Part model, mm, in its own coordinate system. A direction names the side the tool comes from. Round coordinates to 2 decimals unless told otherwise and drop trailing zeros. Order: outer loops, then holes, each group sorted by start corner. A loop starts at its lowest first (then second) coordinate and runs counter-clockwise, first axis right, second up. Notation, with made-up numbers: (25.5, 14.5) -> (49.5, 14.5) arc R14 ccw to (49.5, 23.5) -> close; hole circle Ø10 at (53, -12). An arc over 180 degrees is marked (long way). Answer as a JSON object with one key per item and string values. Group by question number.
```python
from build123d import *

# Parameters (mm, degrees)
SKETCH1_R             = 2.6
BOSS_EXTRUDE1_DEPTH   = 1.6
SKETCH2_R             = 3.45
BOSS_EXTRUDE2_DEPTH   = 1.4
M5X0_8_TAPPED_HOLE1_D = 4.2


with BuildPart() as part:
    # Sketch1 → Boss-Extrude1 (new body)
    with BuildSketch(Plane.XY):
        with BuildLine():
            Line((-10, -8.5), (-10, 8.5))
            ThreePointArc((-10, 8.5), (-9.560660172, 9.560660172), (-8.5, 10))
            Line((-8.5, 10), (-5, 10))
            Line((-5, 10), (-5, 37.485))
            Line((-5, 37.485), (-3.841886117, 40.959341649))
            ThreePointArc((-3.841886117, 40.959341649), (-3.295926597, 41.701863278), (-2.41886117, 41.985))
            Line((-2.41886117, 41.985), (2.41886117, 41.985))
            ThreePointArc((2.41886117, 41.985), (3.295926597, 41.701863278), (3.841886117, 40.959341649))
            Line((3.841886117, 40.959341649), (5, 37.485))
            Line((5, 37.485), (5, 10))
            Line((5, 10), (8.5, 10))
            ThreePointArc((8.5, 10), (9.560660172, 9.560660172), (10, 8.5))
            Line((10, 8.5), (10, -8.5))
            ThreePointArc((10, -8.5), (9.560660172, -9.560660172), (8.5, -10))
            Line((8.5, -10), (5, -10))
            Line((5, -10), (5, -37.485))
            Line((5, -37.485), (3.841886117, -40.959341649))
            ThreePointArc((3.841886117, -40.959341649), (3.295926597, -41.701863278), (2.41886117, -41.985))
            Line((2.41886117, -41.985), (-2.41886117, -41.985))
            ThreePointArc((-2.41886117, -41.985), (-3.295926597, -41.701863278), (-3.841886117, -40.959341649))
            Line((-3.841886117, -40.959341649), (-5, -37.485))
            Line((-5, -37.485), (-5, -10))
            Line((-5, -10), (-8.5, -10))
            ThreePointArc((-8.5, -10), (-9.560660172, -9.560660172), (-10, -8.5))
        make_face()
        Circle(SKETCH1_R, mode=Mode.SUBTRACT)
    extrude(amount=BOSS_EXTRUDE1_DEPTH)

    # Sketch2 → Boss-Extrude2 (add)
    with BuildSketch(Plane.XY.offset(1.6)):
        with Locations((0, 14.95)):
            Circle(SKETCH2_R)
        with Locations((0, 34.95)):
            Circle(SKETCH2_R)
        with Locations((0, -14.95)):
            Circle(SKETCH2_R)
        with Locations((0, -34.95)):
            Circle(SKETCH2_R)
    extrude(amount=BOSS_EXTRUDE2_DEPTH)

    # M5x0.8 Tapped Hole1 (through all)
    with Locations(Plane.XY.offset(3)):
        with Locations((0, 34.95), (0, 14.95), (0, -14.95), (0, -34.95)):
            Hole(M5X0_8_TAPPED_HOLE1_D / 2)


solid = part.part
```
Q1. Band-saw the part on B-B (y = -34.95). List the corners of the cut face in (x, z).
Q2. Wall check: line 1 (Y direction, x = 0, z = 0.7) (3 decimals); line 2 (X direction, y = 35, z = 0.1); line 3 (Z direction, x = 3.25, y = 19.5). Give the ranges that are in metal, low to high. Write a range as [from, to].
Q3. Drop flat-ended pins along their axis: pin 1 Ø4 at (x, y) = (0, 0) entering from +Z; pin 2 Ø10 at (x, y) = (-3.5, 4.5) entering from +Z; pin 3 Ø0.5 at (x, z) = (6.5, 1) entering from +Y; pin 4 Ø0.8 at (y, z) = (-29.5, 1) entering from -X. Give the stop position or say it passes through.
Q4. Band-saw the part on A-A (z = 2.45). List the corners of the cut face in (x, y), plus the area to 3 significant figures.
Q5. Band-saw the part on C-C (x = 6.5). List the corners of the cut face in (y, z).
Q6. Which spindle directions (+Z, -Z, +X, -X, +Y, -Y) get a long thin tool onto all of the face, cutting with end or side? Do faces 1 (the flat face through (-0.05, -17.2, 3)), 2 (the flat face through (-7, -10, 1)), 3 (the flat face through (7, -10, 1)), 4 (the flat face through (7, 10, 1)), 5 (the cylindrical face through (-0.45, 38.37, 2.29)). Say none if no direction does.
Q7. Two-plate mould, pull along Y, no slides. Class faces 6 (the cylindrical face through (-0.338, 2.578, 0.789)), 7 (the cylindrical face through (-1.13, 16.72, 1.48)), 8 (the cylindrical face through (9.55, 9.57, 0.79)), 9 (the flat face through (-5, -24, 1)): +Y half, -Y half, draft (parallel to the pull), parting line (faces both ways), or undercut.
Q8. Band-saw the part on D-D (y = 0). List the corners of the cut face in (x, z).
Completed:
{
 "1": {"outline": "(-5, 0) -> (-2.1, 0) -> (-2.1, 3) -> (-3.45, 3) -> (-3.45, 1.6) -> (-5, 1.6) -> close; (2.1, 0) -> (5, 0) -> (5, 1.6) -> (3.45, 1.6) -> (3.45, 3) -> (2.1, 3) -> close"},
 "2": {"line 1": "[-41.985, -37.05], [-32.85, -17.05], [-12.85, -2.6], [2.6, 12.85], [17.05, 32.85], [37.05, 41.985]", "line 2": "[-5, -2.1], [2.1, 5]", "line 3": "[0, 1.6]"},
 "3": {"pin 1": "through", "pin 2": "z = 1.6", "pin 3": "y = 10", "pin 4": "x = -5"},
 "4": {"outline": "circle Ø6.9 at (0, -34.95); circle Ø6.9 at (0, -14.95); circle Ø6.9 at (0, 14.95); circle Ø6.9 at (0, 34.95); hole circle Ø4.2 at (0, -34.95); hole circle Ø4.2 at (0, -14.95); hole circle Ø4.2 at (0, 14.95); hole circle Ø4.2 at (0, 34.95)", "area": "94.2 mm2"},
 "5": {"outline": "(-10, 0) -> (10, 0) -> (10, 1.6) -> (-10, 1.6) -> close"},
 "6": {"face 1": "+Z, +X, -X, +Y, -Y", "face 2": "+Z, -Z, -X, -Y", "face 3": "+Z, -Z, +X, -Y", "face 4": "+Z, -Z, +X, +Y", "face 5": "+Z"},
 "7": {"face 6": "undercut", "face 7": "undercut", "face 8": "+Y half", "face 9": "draft"},
 "8": {"outline": "(-10, 0) -> (-2.6, 0) -> (-2.6, 1.6) -> (-10, 1.6) -> close; (2.6, 0) -> (10, 0) -> (10, 1.6) -> (2.6, 1.6) -> close"}
}
